from build123d import *

# Parameters (mm, degrees)
EXTRUDE_1_DEPTH      = 25
CUT_EXTRUDE_4_DEPTH  = 80.457942189
SKETCH_7_W           = 16.60831278
SKETCH_7_H           = 38.473598513
CUT_EXTRUDE_14_DEPTH = 80.457942189
SKETCH_8_W           = 5
SKETCH_8_H           = 30.968526609
EXTRUDE_2_DEPTH      = 25
EXTRUDE_3_DEPTH      = 25
FILLET_4_R           = 1
SKETCH_10_W          = 10.885979968
SKETCH_10_H          = 16.094938527
CUT_EXTRUDE_15_DEPTH = 80.457942189
SKETCH_11_W          = 4.5
SKETCH_11_H          = 22
EXTRUDE_5_DEPTH      = 25
SKETCH_14_W          = 45
SKETCH_14_H          = 4
EXTRUDE_6_DEPTH      = 25
SKETCH_15_R          = 3.25
CUT_EXTRUDE_19_DEPTH = 10
FILLET_5_R           = 12.5
FILLET_6_R           = 3
FILLET_7_R           = 7
FILLET_8_R           = 3
SKETCH_17_W          = 2
SKETCH_17_H          = 5
CUT_EXTRUDE_21_DEPTH = 23


with BuildPart() as part:
    # Эскиз1 → Бобышка-Вытянуть1 (new body)
    with BuildSketch(Plane(origin=(0, 0, 0), x_dir=(1, 0, 0), z_dir=(0, 1, 0))):
        Polygon((-66.825757576, 34.969739794), (-66.825757576, 29.969739794), (-63.825757576, 29.969739794), (-63.825757576, 31.969739794), (-38.825757576, 31.969739794), (-38.825757576, 6.969739794), (-63.825757576, 6.969739794), (-63.825757576, 8.969739794), (-66.825757576, 8.969739794), (-66.825757576, 3.969739794), (-22.123470102, 3.969739794), (-36.579007505, 34.969739794), align=None)
    extrude(amount=EXTRUDE_1_DEPTH)

    # Эскиз3 → Вырез-Вытянуть4 (cut, through all)
    with BuildSketch(Plane.XZ):
        Polygon((-66.825757576, -3.969739794), (-65.325757576, -8.969739794), (-66.825757576, -8.969739794), align=None)
        Polygon((-66.825757576, -29.969739794), (-66.825757576, -34.969739794), (-65.325757576, -29.969739794), align=None)
    extrude(amount=-CUT_EXTRUDE_4_DEPTH, mode=Mode.SUBTRACT)

    # Эскиз7 → Вырез-Вытянуть14 (cut, through all)
    with BuildSketch(Plane(origin=(0, 0, 0), x_dir=(-1, 0, 0), z_dir=(0, -1, 0))):
        with Locations((27.703474463, 20.539743139)):
            Rectangle(SKETCH_7_W, SKETCH_7_H)
    extrude(amount=-CUT_EXTRUDE_14_DEPTH, mode=Mode.SUBTRACT)

    # Эскиз8 → Бобышка-Вытянуть2 (add)
    with BuildSketch(Plane(origin=(0, 0, 0), x_dir=(-1, 0, 0), z_dir=(0, -1, 0))):
        with Locations((36.298943925, 19.454003098)):
            Rectangle(SKETCH_8_W, SKETCH_8_H)
    extrude(amount=-EXTRUDE_2_DEPTH)

    # Эскиз9 → Бобышка-Вытянуть3 (add)
    with BuildSketch(Plane.XZ):
        with BuildLine():
            Line((-25.798943925, -9.121669553), (-24.000865345, -7.695483003))
            ThreePointArc((-24.000865345, -7.695483003), (-36.096342696, -11.954003099), (-24.000865345, -16.212523195))
            Line((-24.000865345, -16.212523195), (-25.798943925, -14.786336644))
            ThreePointArc((-25.798943925, -14.786336644), (-33.80140029, -11.954003099), (-25.798943925, -9.121669553))
        make_face()
        with BuildLine():
            Line((-25.798943925, -24.130682885), (-24.000865345, -22.7126007))
            ThreePointArc((-24.000865345, -22.7126007), (-36.0856317, -26.954003099), (-24.000865345, -31.195405497))
            Line((-24.000865345, -31.195405497), (-25.798943925, -29.777323313))
            ThreePointArc((-25.798943925, -29.777323313), (-33.795735785, -26.954003099), (-25.798943925, -24.130682885))
        make_face()
    extrude(amount=-EXTRUDE_3_DEPTH)

    # Скругление4
    fillet_4_edges = [part.edges().sort_by_distance(p)[0] for p in [
        (-24.000865345, 12.5, -7.695483003),
        (-24.000865345, 12.5, -16.212523195),
        (-24.000865345, 12.5, -22.7126007),
        (-24.000865345, 12.5, -31.195405497),
    ]]
    fillet(fillet_4_edges, radius=FILLET_4_R)

    # Эскиз10 → Вырез-Вытянуть15 (cut, through all)
    with BuildSketch(Plane(origin=(0, 25, 0), x_dir=(1, 0, 0), z_dir=(0, 1, 0))):
        with Locations((-28.355953941, 12.017209058)):
            Rectangle(SKETCH_10_W, SKETCH_10_H)
    extrude(amount=-CUT_EXTRUDE_15_DEPTH, mode=Mode.SUBTRACT)

    # Эскиз11 → Бобышка-Вытянуть5 (add)
    with BuildSketch(Plane(origin=(0, 25, 0), x_dir=(1, 0, 0), z_dir=(0, 1, 0))):
        with Locations((-31.548943925, 42.450794958)):
            Rectangle(SKETCH_11_W, SKETCH_11_H)
    extrude(amount=-EXTRUDE_5_DEPTH)

    # Эскиз14 → Бобышка-Вытянуть6 (add)
    with BuildSketch(Plane(origin=(0, 25, 0), x_dir=(1, 0, 0), z_dir=(0, 1, 0))):
        with Locations((-11.298943925, 51.450794958)):
            Rectangle(SKETCH_14_W, SKETCH_14_H)
    extrude(amount=-EXTRUDE_6_DEPTH)

    # Эскиз15 → Вырез-Вытянуть19 (cut)
    with BuildSketch(Plane(origin=(0, 0, -53.450794958), x_dir=(-1, 0, 0), z_dir=(0, 0, -1))):
        with Locations((1.298943925, 12.5)):
            Circle(SKETCH_15_R)
    extrude(amount=-CUT_EXTRUDE_19_DEPTH, mode=Mode.SUBTRACT)

    # Скругление5
    fillet_5_edges = [part.edges().sort_by_distance(p)[0] for p in [
        (11.201056075, 0, -51.450794958),
        (11.201056075, 25, -51.450794958),
    ]]
    fillet(fillet_5_edges, radius=FILLET_5_R - 0.0001)  # a hair under: the kernel refuses the full size

    # Скругление6
    fillet_6_edges = [part.edges().sort_by_distance(p)[0] for p in [
        (-29.298943925, 12.5, -49.450794958),
    ]]
    fillet(fillet_6_edges, radius=FILLET_6_R)

    # Скругление7
    fillet_7_edges = [part.edges().sort_by_distance(p)[0] for p in [
        (-33.798943925, 12.5, -53.450794958),
    ]]
    fillet(fillet_7_edges, radius=FILLET_7_R)

    # Скругление8
    fillet_8_edges = [part.edges().sort_by_distance(p)[0] for p in [
        (-33.798943925, 12.5, -21.873734311),
        (-29.298943925, 12.5, -33.740690873),
    ]]
    fillet(fillet_8_edges, radius=FILLET_8_R)

    # Эскиз17 → Вырез-Вытянуть21 (cut)
    with BuildSketch(Plane.XY.offset(-3.969739794)):
        with Locations((-32.798943925, 17.5)):
            Rectangle(SKETCH_17_W, SKETCH_17_H)
        with Locations((-32.798943925, 7.5)):
            Rectangle(SKETCH_17_W, SKETCH_17_H)
    extrude(amount=-CUT_EXTRUDE_21_DEPTH, mode=Mode.SUBTRACT)


solid = part.part
Build history of the part. All positions in model axes, mm. A direction names the side the tool comes from. Give positions to 0.01 mm unless a question says otherwise; leave off trailing zeros. Write each loop counter-clockwise with the first axis right and the second up, starting at its lowest first coordinate (ties: lowest second). Pieces come first, ordered by that corner, then holes. Notation, with made-up numbers: (-36, -30) - (-28, -30) arc R18 ccw to (-28, -2) - close; hole circle Ø10 at (19, 8.5). An arc over 180 degrees is marked (long way). Use one line per item in the form item = value. Start each with the question number.
1. Drop flat-ended pins along their axis: pin 1 Ø0.6 at (y, z) = (12, -31) entering from +X; pin 2 Ø2.5 at (y, z) = (8.5, -21.5) entering from -X; pin 3 Ø7.5 at (x, y) = (0, 16) entering from +Z; pin 4 Ø5 at (x, y) = (-1.3, 12.5) entering from +Z. Give the stop position or say it passes through.
2. Band-saw the part on A-A on x = -55. Write the cut outline in (y, z), plus the area to 3 significant figures.
3. Band-saw the part on C-C on z = -44.5. Write the cut outline in (x, y), plus the area to 4 significant figures.
4. 3-axis set-ups, long thin cutter, end or side, ignore diameter. For faces 1 (the face through (-51, 12, -6.97)), 2 (the face through (-65, 12, -8.97)), 3 (the face through (-28.739, 12.325, -34.524)): which of +Z, -Z, +X, -X, +Y, -Y reach the whole face in a straight line?
5. Probe line 1 (Z direction, x = 4, y = 8.25); line 2 (X direction, y = 18.75, z = -40.5); line 3 (Z direction, x = -58.5, y = 14.75). List the from-to ranges inside material, lowest first. Write a range as [from, to].
6. Two-plate mould, pull along X, no slides. Class faces 4 (the face through (-29.299, 13, -41)), 5 (the face through (-27.36, 12.32, -20.45)): released by +X, released by -X, zero draft, split by the parting line, or undercut.
Conclusion:
q1.pin_1 = -24.48
q1.pin_2 = -38.83
q1.pin_3 = -49.45
q1.pin_4 = through
q2.outline = (0, -34.97) - (25, -34.97) - (25, -31.97) - (0, -31.97) - close; (0, -6.97) - (25, -6.97) - (25, -3.97) - (0, -3.97) - close
q2.area = 150 mm²
q3.outline = (-33.8, 0) - (-29.3, 0) - (-29.3, 25) - (-33.8, 25) - close
q3.area = 112.5 mm²
q4.face_1 = +Y, -Y
q4.face_2 = -X, +Y, -Y
q4.face_3 = +X, +Y, -Y
q5.line_1 = [-53.45, -49.45]
q5.line_2 = [-33.8, -29.3]
q5.line_3 = [-34.97, -31.97], [-6.97, -3.97]
q6.face_4 = released by +X
q6.face_5 = undercut
